Drawing for the job (mm, zero at the part's lowest x, y, z). Round coordinates to 2 decimals unless told otherwise and drop trailing zeros. Order: outer loops, then holes, each group sorted by start corner. A loop starts at its lowest first (then second) coordinate and runs counter-clockwise, first axis right, second up. Notation, with made-up numbers: (74.5, 57.25) - (86.5, 57.25) arc R24 ccw to (86.5, 94.25) - close; hole circle Ø3 at (-21, 30). An arc over 180 degrees is marked (long way). Answer as a JSON object with one key per item and string values.
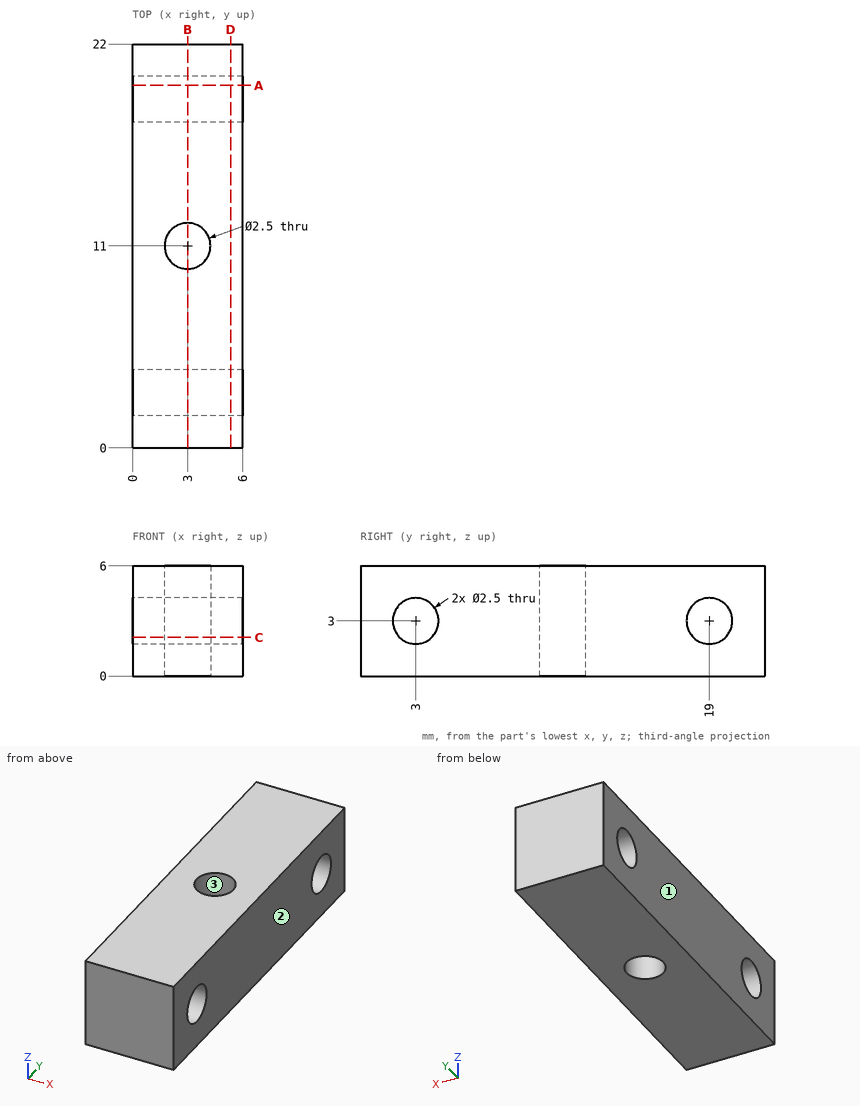
Item 1: Cut at C-C (z = 2.1). Write the cut outline in (x, y).
Taken from the geometry:
{"outline": "(0, 0) - (6, 0) - (6, 2.13) - (0, 2.13) - close; (0, 3.87) - (6, 3.87) - (6, 18.13) - (0, 18.13) - close; (0, 19.87) - (6, 19.87) - (6, 22) - (0, 22) - close; hole circle Ø2.5 at (3, 11)"}
Item 2: Cut at A-A (y = 19.75). Write the cut outline in (x, z).
Taken from the geometry:
{"outline": "(0, 0) - (6, 0) - (6, 2) - (0, 2) - close; (0, 4) - (6, 4) - (6, 6) - (0, 6) - close"}
Item 3: Cut at B-B (x = 3). Write the cut outline in (y, z).
Taken from the geometry:
{"outline": "(0, 0) - (9.75, 0) - (9.75, 6) - (0, 6) - close; (12.25, 0) - (22, 0) - (22, 6) - (12.25, 6) - close; hole circle Ø2.5 at (3, 3); hole circle Ø2.5 at (19, 3)"}
Item 4: Two-plate mould, pull along X, no slides. Class the marked faces 1, 2 and 3: pulls with the +X half, pulls with the -X half, needs draft (parallel to the pull), parting line crosses it, or undercut.
Taken from the geometry:
{"face 1": "pulls with the -X half", "face 2": "pulls with the +X half", "face 3": "undercut"}
Item 5: Probe L1, parallel to Y at x = 2.95, z = 3; L2, parallel to Y at x = 1.7, z = 3; L3, parallel to Y at x = 3, z = 1.7. List the from-to ranges inside material, lowest first. Write a range as from..to.
Taken from the geometry:
{"L1": "0..1.75, 4.25..9.75, 12.25..17.75, 20.25..22", "L2": "0..1.75, 4.25..17.75, 20.25..22", "L3": "0..9.75, 12.25..22"}
Item 6: Drop a flat-ended pin along its axis: P1, Ø2, axis at y = 3, z = 3, coming from the -X side. Give the stop position or say it passes through.
Taken from the geometry:
{"P1": "through"}
Item 7: Cut at D-D (x = 5.35). Write the cut outline in (y, z), plus the area to 3 significant figures.
Taken from the geometry:
{"outline": "(0, 0) - (22, 0) - (22, 6) - (0, 6) - close; hole circle Ø2.5 at (3, 3); hole circle Ø2.5 at (19, 3)", "area": "122 mm2"}
